CAD build for the part. Positions are in the model's coordinates, mm. Face numbers are marked on the shaded views. A direction names the side the tool comes from. Give positions to 0.01 mm unless a question says otherwise; leave off trailing zeros. Loops run counter-clockwise (first coordinate to the right, second up) from the corner with the lowest first, then second, coordinate; pieces in that order, holes last. Notation, with made-up numbers: M 69,65 L 111,65 A22 cw 111,91 Z; hole C 70,-15 d4. An arc over 180 degrees is marked long. Answer as CSV lines item,"result".
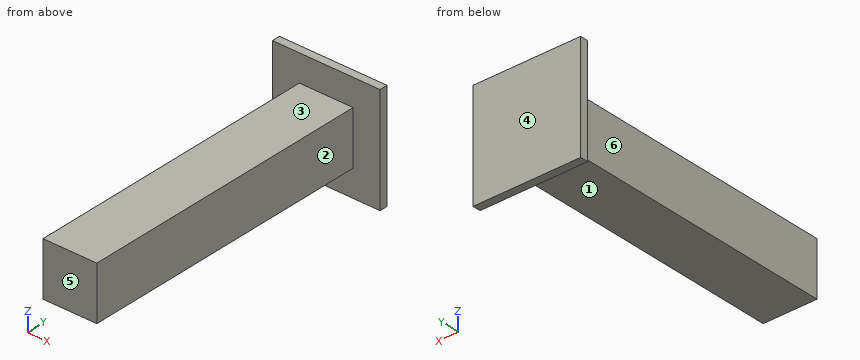
Autodesk Inventor part; units mm, degrees
ref_plane "YZ Plane" through (0, 0, 0) normal (1, 0, 0) x (0, 1, 0)
ref_plane "XZ Plane" through (0, 0, 0) normal (0, 1, 0) x (-1, 0, 0)
ref_plane "XY Plane" through (0, 0, 0) normal (0, 0, 1) x (1, 0, 0)
sketch "Sketch1" plane through (0, 0, 0) normal (0, 1, 0) x (-1, 0, 0)
  line L0 (0, 0) -> (20, 0)
  line L1 (20, 0) -> (20, -20)
  line L2 (20, -20) -> (0, -20)
  line L3 (0, -20) -> (0, 0)
  dimension "d0" = 20
  dimension "d1" = 20
extrude "Extrusion1" add sketch "Sketch1" along normal blind 110
ref_plane "Work Plane1" through (-20, 110, -10) normal (0, 1, 0) x (1, 0, 0)
sketch "Sketch3" plane through (-20, 110, -10) normal (0, 1, 0) x (1, 0, 0)
  line L0 (0, -10) -> (20, -10)
  line L1 (20, -10) -> (20, 10)
  line L2 (30, -20) -> (-10, -20)
  line L3 (-10, -20) -> (-10, 20)
  line L4 (-10, 20) -> (30, 20)
  line L5 (30, 20) -> (30, -20)
  line L6 (30, -20) -> (-10, 20) construction
  line L7 (-10, -20) -> (30, 20) construction
  point P0 (10, 0)
  dimension "d4" = 10
  dimension "d5" = 10
  dimension "d6" = 40
  dimension "d7" = 40
extrude "Extrusion2" add sketch "Sketch3" along normal blind 3
properties part number "TagPillar"
1) Which spindle directions (+Z, -Z, +X, -X, +Y, -Y) get a long thin tool onto all of the face, cutting with end or side? Do the marked faces 1, 2 and 3. Say none if no direction does.
Answer below:
face 1,"-Z, +X, -X, -Y"
face 2,"+Z, -Z, +X, -Y"
face 3,"+Z, +X, -X, -Y"
2) Flat gauge pins, fed straight in: pin 1 (10 mm diameter, centred on x = -12.5, y = 71, fed in from -Z); pin 2 (6 mm diameter, centred on x = -11, y = 37, fed in from +Z); pin 3 (12 mm diameter, centred on y = 84, z = -2, fed in from -X); pin 4 (2 mm diameter, centred on x = -9, z = -4, fed in from -Y). Where does each tip first touch, or does it go through?
Answer below:
pin 1,"stops at z = -20"
pin 2,"stops at z = 0"
pin 3,"stops at x = -20"
pin 4,"stops at y = 0"
3) Band-saw the part on C-C on y = 33.5. Give the cut face in (x, z), and give its area (3 significant figures).
Answer below:
outline,"M -20,-20 L 0,-20 L 0,0 L -20,0 Z"
area,"400 mm^2"
4) Drill centre lines: line 1 (Y direction, x = 8.5, z = -1); line 2 (X direction, y = 32, z = -12.5). Where is each one in solid material? Low to high. Write a range as from..to.
Answer below:
line 1,"y = 110..113"
line 2,"x = -20..0"
5) Band-saw the part on B-B on z = -12. Give the cut face in (x, y).
Answer below:
outline,"M -30,110 L -20,110 L -20,0 L 0,0 L 0,110 L 10,110 L 10,113 L -30,113 Z"
6) Mould opens along Y. For the marked faces 4, 5 and 6 say: +Y half, -Y half, draft (parallel to the pull), parting line (faces both ways), or undercut.
Answer below:
face 4,"+Y half"
face 5,"-Y half"
face 6,"draft"
7) Band-saw the part on A-A on x = -18. Give the cut face in (y, z), and give its area (3 significant figures).
Answer below:
outline,"M 0,-20 L 110,-20 L 110,-30 L 113,-30 L 113,10 L 110,10 L 110,0 L 0,0 Z"
area,"2,320 mm^2"
8) Band-saw the part on D-D on x = 7.5. Give the cut face in (y, z), and give its area (3 significant figures).
Answer below:
outline,"M 110,-30 L 113,-30 L 113,10 L 110,10 Z"
area,"120 mm^2"
